Could you check a few things on this model? Use its own coordinates, in mm. Round coordinates to 2 decimals unless told otherwise and drop trailing zeros. Write each loop counter-clockwise with the first axis right and the second up, starting at its lowest first coordinate (ties: lowest second). Pieces come first, ordered by that corner, then holes. Notation, with made-up numbers: (-1.5, 63) - (20.5, 63) arc R33 cw to (20.5, 97) - close; hole circle Ø6 at (82, 87.5). An arc over 180 degrees is marked (long way). Put each result on its own line as item: value.
Autodesk Inventor part; units mm, degrees
ref_plane "YZ Plane" through (0, 0, 0) normal (1, 0, 0) x (0, 1, 0)
ref_plane "XZ Plane" through (0, 0, 0) normal (0, 1, 0) x (-1, 0, 0)
ref_plane "XY Plane" through (0, 0, 0) normal (0, 0, 1) x (1, 0, 0)
sketch "Sketch1" plane through (0, 0, 0) normal (0, 0, 1) x (1, 0, 0)
  circle A0 centre (0, 0) radius 95
  line L0 (43, 43) -> (-43, 43)
  line L1 (-43, 43) -> (-43, -43)
  line L2 (-43, -43) -> (43, -43)
  line L3 (43, -43) -> (43, 43)
  line L4 (43, 43) -> (-43, -43) construction
  line L5 (-43, 43) -> (43, -43) construction
  dimension "d157" = 190
  dimension "d158" = 86
  dimension "d159" = 86
extrude "Plate5" add sketch "Sketch1" along normal blind 3
sketch "Sketch7" plane through (0, 0, 0) normal (0, 0, -1) x (-1, 0, 0)
  circle A0 centre (0, 80) radius 8.5
  point P0 (0, 0)
  dimension "d160" = 17
  dimension "d161" = 80
extrude "Cut1" cut sketch "Sketch7" against normal blind 3
pattern_circular "Circular Pattern1" count 4 over 360 about axis through (0, 0, -10) along (0, 0, 1) of "Cut1"
chamfer "Corner Chamfer2" distance 25 angle 45 4 edges at (-43, -43, 1.5) (43, -43, 1.5) (-43, 43, 1.5) (43, 43, 1.5)
properties part number "TZS 0972 funnel FLANGE 50-90" material "Stainless Steel"
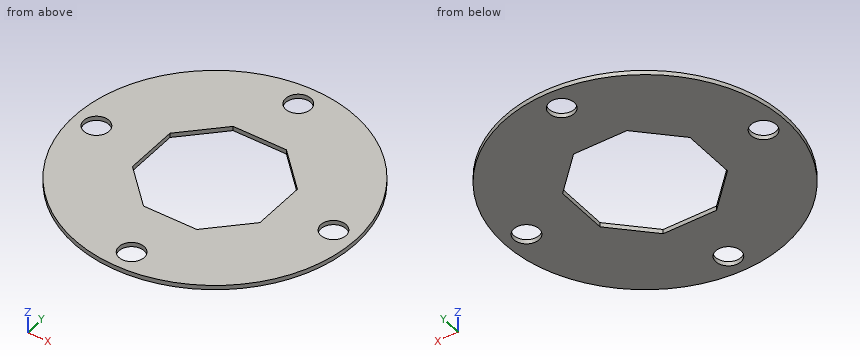
(1) Imagine slicing it at B-B, the plane z = 2.1. List the corners of the cut face in (x, y) for me, then the cut area to 3 significant figures.
Values found:
outline: circle Ø190 at (0, 0); hole circle Ø17 at (-80, 0); hole (-43, -18) - (-18, -43) - (18, -43) - (43, -18) - (43, 18) - (18, 43) - (-18, 43) - (-43, 18) - close; hole circle Ø17 at (0, -80); hole circle Ø17 at (0, 80); hole circle Ø17 at (80, 0)
area: 21,300 mm^2
(2) Please list where these lines run through material, in increasing order: probe 1 along Y at (x, z) = (0, 0.7); probe 2 along Y at (x, z) = (-80, 1.1); probe 3 along Y at (x, z) = (-38, 1.8). Write a range as from..to.
Values found:
probe 1: y = -95..-88.5, -71.5..-43, 43..71.5, 88.5..95
probe 2: y = -51.23..-8.5, 8.5..51.23
probe 3: y = -87.07..-23, 23..87.07
(3) I'm going to push flat-ended pins straight in: pin 1 (1.5 mm diameter, centred on y = 24, z = 2.5, fed in from -X); pin 2 (1 mm diameter, centred on y = -73.5, z = 0.5, fed in from -X); pin 3 (1 mm diameter, centred on x = 19, z = 1.5, fed in from +Y). Where does each tip first touch, or does it pass through?
Values found:
pin 1: stops at x = -92.11
pin 2: stops at x = -60.79
pin 3: stops at y = 93.18
(4) Imagine slicing it at D-D, the plane x = -80. List the corners of the cut face in (y, z) for me, then the cut area to 3 significant figures.
Values found:
outline: (-51.23, 0) - (-8.5, 0) - (-8.5, 3) - (-51.23, 3) - close; (8.5, 0) - (51.23, 0) - (51.23, 3) - (8.5, 3) - close
area: 256 mm^2
(5) Imagine slicing it at A-A, the plane y = 0. List the corners of the cut face in (x, z) for me.
Values found:
outline: (-95, 0) - (-88.5, 0) - (-88.5, 3) - (-95, 3) - close; (-71.5, 0) - (-43, 0) - (-43, 3) - (-71.5, 3) - close; (43, 0) - (71.5, 0) - (71.5, 3) - (43, 3) - close; (88.5, 0) - (95, 0) - (95, 3) - (88.5, 3) - close
